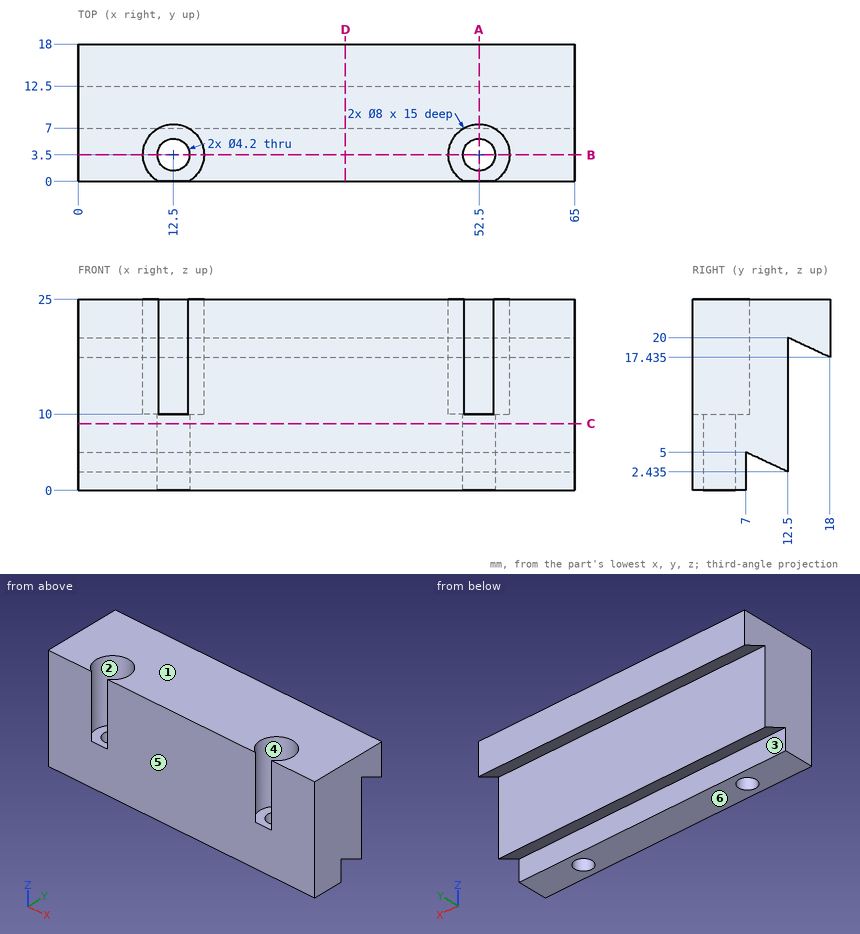
Source: three-view drawing plus pictorial views. Frame: mm from the lowest corner of the part. A direction names the side the tool comes from. Coordinates: 2 decimals unless noted, no trailing zeros. Loops run counter-clockwise (first coordinate to the right, second up) from the corner with the lowest first, then second, coordinate; pieces in that order, holes last. Notation, with made-up numbers: (70.25, -28.75) -> (106.25, -28.75) arc R21 cw to (106.25, -12.75) -> close; hole circle Ø9 at (30.25, 57). An arc over 180 degrees is marked (long way). One line per item, written item: value.
(1) Cut plane B-B (y = 3.5). Output: boundary loops of the cut face in (x, z).
Answer below:
outline: (0, 0) -> (10.4, 0) -> (10.4, 10) -> (8.5, 10) -> (8.5, 25) -> (0, 25) -> close; (14.6, 0) -> (50.4, 0) -> (50.4, 10) -> (48.5, 10) -> (48.5, 25) -> (16.5, 25) -> (16.5, 10) -> (14.6, 10) -> close; (54.6, 0) -> (65, 0) -> (65, 25) -> (56.5, 25) -> (56.5, 10) -> (54.6, 10) -> close
(2) Set-up query: the marked faces 1, 2 and 3. Return all of +Z, -Z, +X, -X, +Y, -Y with unobstructed straight access to the full face (end or side cutting, diameter ignored); none if empty.
Answer below:
face 1: +Z, +X, -X, +Y, -Y
face 2: +Z
face 3: -Z, +X, -X
(3) Pin query (flat end, axial travel): pin 1 Ø1.5 at (y, z) = (15, 5) entering from -X; pin 2 Ø2 at (x, y) = (14, 3) entering from +Z; pin 3 Ø2.5 at (x, z) = (23, 2) entering from +Y. Return the tip coordinate at first contact, or that it passes through.
Answer below:
pin 1: passes through
pin 2: stops at z = 10
pin 3: stops at y = 12.5
(4) Draft query along Y for the marked faces 4, 5 and 6. Return one class per face: pulls with the +Y half, pulls with the -Y half, needs draft (parallel to the pull), parting line crosses it, or undercut.
Answer below:
face 4: undercut
face 5: pulls with the -Y half
face 6: needs draft
(5) Cut plane A-A (x = 52.5). Output: boundary loops of the cut face in (y, z) (1 decimal).
Answer below:
outline: (0, 0) -> (1.4, 0) -> (1.4, 10) -> (0, 10) -> close; (5.6, 0) -> (7, 0) -> (7, 5) -> (12.5, 2.4) -> (12.5, 20) -> (18, 17.4) -> (18, 25) -> (7.5, 25) -> (7.5, 10) -> (5.6, 10) -> close
(6) Cut plane D-D (x = 35). Output: boundary loops of the cut face in (y, z) (1 decimal), then the cut area to 3 significant figures.
Answer below:
outline: (0, 0) -> (7, 0) -> (7, 5) -> (12.5, 2.4) -> (12.5, 20) -> (18, 17.4) -> (18, 25) -> (0, 25) -> close
area: 327 mm2
(7) Ray query, line 1 along X through (y, z) = (3.5, 15.75); line 2 along X through (y, z) = (4.75, 8); line 3 along Y through (x, z) = (10, 1.5). Return the intervals inside material, ascending.
Answer below:
line 1: x = 0 to 8.5, 16.5 to 48.5, 56.5 to 65
line 2: x = 0 to 10.81, 14.19 to 50.81, 54.19 to 65
line 3: y = 0 to 7
(8) Cut plane C-C (z = 8.75). Output: boundary loops of the cut face in (x, y), then the cut area to 3 significant figures.
Answer below:
outline: (0, 0) -> (65, 0) -> (65, 12.5) -> (0, 12.5) -> close; hole circle Ø4.2 at (12.5, 3.5); hole circle Ø4.2 at (52.5, 3.5)
area: 785 mm2
